from build123d import *

# Parameters (mm, degrees)
SKETCH1_W           = 100
SKETCH1_H           = 85
BOSS_EXTRUDE1_DEPTH = 30
SKETCH3_R           = 2.5
CUT_EXTRUDE1_DEPTH  = 50
SKETCH4_R           = 4
CUT_EXTRUDE2_DEPTH  = 20
CUT_EXTRUDE5_DEPTH  = 25
SKETCH8_R           = 7.5
CUT_EXTRUDE6_DEPTH  = 31


with BuildPart() as part:
    # Sketch1 → Boss-Extrude1 (new body)
    with BuildSketch(Plane.XY):
        Rectangle(SKETCH1_W, SKETCH1_H)
    extrude(amount=BOSS_EXTRUDE1_DEPTH)

    # Sketch3 → Cut-Extrude1 (cut)
    with BuildSketch(Plane.XY.offset(30)):
        with Locations((-43.5, 36)):
            Circle(SKETCH3_R)
        with Locations((43.5, 36)):
            Circle(SKETCH3_R)
        with Locations((43.5, -36)):
            Circle(SKETCH3_R)
        with Locations((-43.5, -36)):
            Circle(SKETCH3_R)
    extrude(amount=-CUT_EXTRUDE1_DEPTH, mode=Mode.SUBTRACT)

    # Sketch4 → Cut-Extrude2 (cut)
    with BuildSketch(Plane.XY.offset(30)):
        with Locations((-43.5, 36)):
            Circle(SKETCH4_R)
        with Locations((43.5, 36)):
            Circle(SKETCH4_R)
        with Locations((-43.5, -36)):
            Circle(SKETCH4_R)
        with Locations((43.5, -36)):
            Circle(SKETCH4_R)
    extrude(amount=-CUT_EXTRUDE2_DEPTH, mode=Mode.SUBTRACT)

    # Sketch7 → Cut-Extrude5 (cut)
    with BuildSketch(Plane(origin=(0, 0, 0), x_dir=(-1, 0, 0), z_dir=(0, 0, -1))):
        with BuildLine():
            Line((-32, 37), (32, 37))
            ThreePointArc((32, 37), (39.071067812, 34.071067812), (42, 27))
            Line((42, 27), (42, -27))
            ThreePointArc((42, -27), (39.071067812, -34.071067812), (32, -37))
            Line((32, -37), (-32, -37))
            ThreePointArc((-32, -37), (-39.071067812, -34.071067812), (-42, -27))
            Line((-42, -27), (-42, 27))
            ThreePointArc((-42, 27), (-39.071067812, 34.071067812), (-32, 37))
        make_face()
    extrude(amount=-CUT_EXTRUDE5_DEPTH, mode=Mode.SUBTRACT)

    # Sketch8 → Cut-Extrude6 (cut, through all)
    with BuildSketch(Plane.XY.offset(30)):
        with Locations((0, -22.5)):
            Circle(SKETCH8_R)
    extrude(amount=-CUT_EXTRUDE6_DEPTH, mode=Mode.SUBTRACT)


solid = part.part
Part model, mm, in its own coordinate system. A direction names the side the tool comes from. Give positions to 0.01 mm unless a question says otherwise; leave off trailing zeros. Write each loop counter-clockwise with the first axis right and the second up, starting at its lowest first coordinate (ties: lowest second). Pieces come first, ordered by that corner, then holes.
1) Cut at B-B on y = -22.5. Write the cut outline in (x, z), then the cut area to 3 significant figures.
Resolved:
outline: (-50, 0) - (-42, 0) - (-42, 25) - (-7.5, 25) - (-7.5, 30) - (-50, 30) - close; (7.5, 25) - (42, 25) - (42, 0) - (50, 0) - (50, 30) - (7.5, 30) - close
area: 825 mm2
2) Which spindle directions (+Z, -Z, +X, -X, +Y, -Y) get a long thin tool onto all of the face, cutting with end or side? Do faces 5 (the face through (-44.021, 39.966, 20.14)), 6 (the face through (-41.115, -35.249, 5.07)), 7 (the face through (-1, 1, 25)). Say none if no direction does.
Resolved:
face 5: +Z
face 6: +Z, -Z
face 7: -Z
3) Cut at D-D on x = -43.5. Write the cut outline in (y, z).
Resolved:
outline: (-42.5, 0) - (-38.5, 0) - (-38.5, 10) - (-40, 10) - (-40, 30) - (-42.5, 30) - close; (-33.5, 0) - (33.5, 0) - (33.5, 10) - (32, 10) - (32, 30) - (-32, 30) - (-32, 10) - (-33.5, 10) - close; (38.5, 0) - (42.5, 0) - (42.5, 30) - (40, 30) - (40, 10) - (38.5, 10) - close
4) Probe L1, parallel to Y at x = 43.5, z = 5.5; L2, parallel to X at y = -16, z = 9.5; L3, parallel to Y at x = 13, z = 8. List the from-to ranges inside material, lowest first.
Resolved:
L1: y = -42.5 to -38.5, -33.5 to 33.5, 38.5 to 42.5
L2: x = -50 to -42, 42 to 50
L3: y = -42.5 to -37, 37 to 42.5
5) Two-plate mould, pull along X, no slides. Class faces 1 (the face through (-41.19, 35.04, 5.07)), 2 (the face through (-1, 42.5, 15)), 3 (the face through (43, 33, 10)), 4 (the face through (-50, -1, 15)): released by +X, released by -X, zero draft, split by the parting line, or undercut.
Resolved:
face 1: undercut
face 2: zero draft
face 3: undercut
face 4: released by -X
6) Cut at A-A on x = 0. Write the cut outline in (y, z).
Resolved:
outline: (-42.5, 0) - (-37, 0) - (-37, 25) - (-30, 25) - (-30, 30) - (-42.5, 30) - close; (-15, 25) - (37, 25) - (37, 0) - (42.5, 0) - (42.5, 30) - (-15, 30) - close
7) Pin check, flat tips, straight feed: pin 1 (9 mm diameter, centred on x = 41.5, y = -34.5, fed in from +Z); pin 2 (1.5 mm diameter, centred on x = -20.5, y = -20.5, fed in from -Z); pin 3 (7 mm diameter, centred on x = -43.5, y = 36, fed in from +Z). Stop position of each tip, or through.
Resolved:
pin 1: stops at z = 30
pin 2: stops at z = 25
pin 3: stops at z = 10
8) Cut at C-C on z = 3.25. Write the cut outline in (x, y), then the cut area to 3 significant figures.
Resolved:
outline: (-50, -42.5) - (50, -42.5) - (50, 42.5) - (-50, 42.5) - close; hole circle Ø5 at (-43.5, -36); hole circle Ø5 at (-43.5, 36); hole (-42, -27) arc R10 ccw to (-32, -37) - (32, -37) arc R10 ccw to (42, -27) - (42, 27) arc R10 ccw to (32, 37) - (-32, 37) arc R10 ccw to (-42, 27) - close; hole circle Ø5 at (43.5, -36); hole circle Ø5 at (43.5, 36)
area: 2,290 mm2
